Design review of the part shown in the three views and the two pictorial views. Dimensions are in mm from the part's minimum x, y and z. Coordinates: 2 decimals unless noted, no trailing zeros. Order: outer loops, then holes, each group sorted by start corner. A loop starts at its lowest first (then second) coordinate and runs counter-clockwise, first axis right, second up. Notation, with made-up numbers: (21, 62) -> (54, 62) arc R28 cw to (54, 89) -> close; hole circle Ø11 at (23.5, 72). An arc over 180 degrees is marked (long way). Answer as a JSON object with one key per item and string values. Group by question number.
1) Draft analysis for pull direction Y (two halves, no side actions). For the marked faces 1, 2, 3 and 4, state which applies: +Y half, -Y half, draft (parallel to the pull), parting line (faces both ways), or undercut.
2) Wall thickness on L1, parallel to Y at x = 3, z = 1.2; L2, parallel to Y at x = 16, z = 1.4; L3, parallel to X at y = 2.5, z = 0.4: over which ranges is each line inside the solid? List them lowest first.
3) Add section A-A, the plane y = 10. Write out the cut boundary in (x, z), then the cut area to 3 significant figures.
4) For pin 1 (2 mm diameter, centred on x = 17, y = 17, fed in from +Z), flat-tipped, find the tip position at first contact; note if it passes through.
5) Add section C-C, the plane y = 17. Write out the cut boundary in (x, z), then the cut area to 3 significant figures.
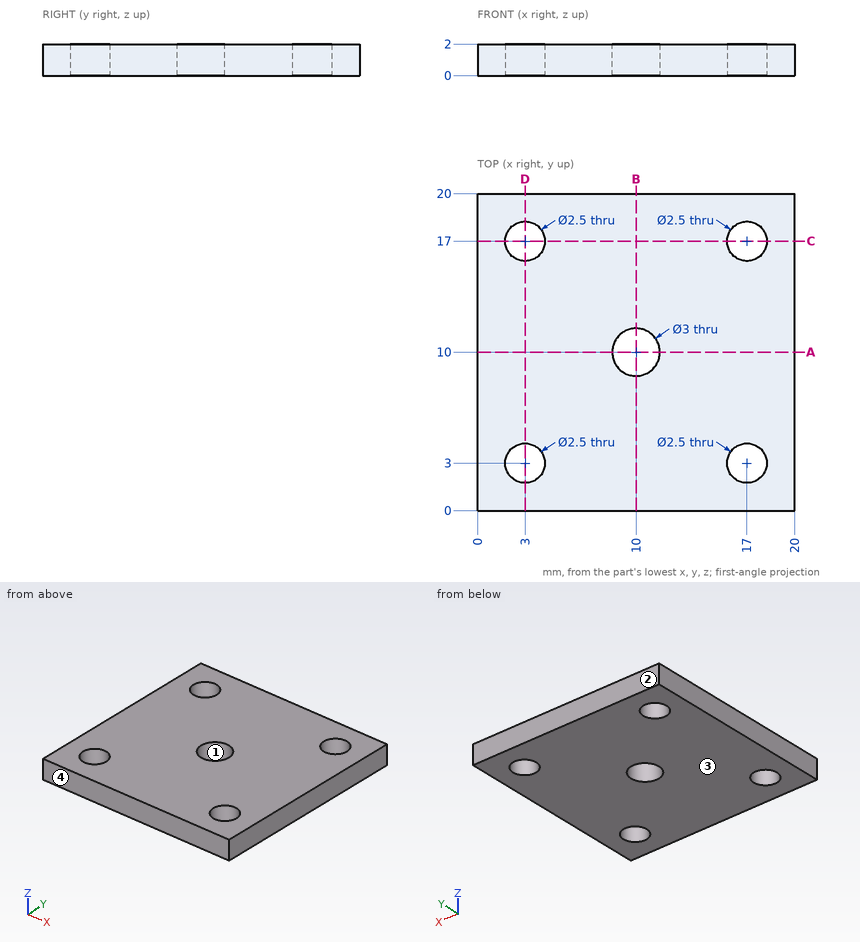
Output values:
{
 "1": {"face 1": "undercut", "face 2": "+Y half", "face 3": "draft", "face 4": "-Y half"},
 "2": {"L1": "y = 0 to 1.75, 4.25 to 15.75, 18.25 to 20", "L2": "y = 0 to 2.25, 3.75 to 16.25, 17.75 to 20", "L3": "x = 0 to 1.85, 4.15 to 15.85, 18.15 to 20"},
 "3": {"outline": "(0, 0) -> (8.5, 0) -> (8.5, 2) -> (0, 2) -> close; (11.5, 0) -> (20, 0) -> (20, 2) -> (11.5, 2) -> close", "area": "34.0 mm²"},
 "4": {"pin 1": "passes through"},
 "5": {"outline": "(0, 0) -> (1.75, 0) -> (1.75, 2) -> (0, 2) -> close; (4.25, 0) -> (15.75, 0) -> (15.75, 2) -> (4.25, 2) -> close; (18.25, 0) -> (20, 0) -> (20, 2) -> (18.25, 2) -> close", "area": "30.0 mm²"}
}
